Geometry check sheet. Reference: drawing and pictorial views, mm from the part's lowest x, y, z. A direction names the side the tool comes from. Coordinates: 2 decimals unless noted, no trailing zeros. Loops run counter-clockwise (first coordinate to the right, second up) from the corner with the lowest first, then second, coordinate; pieces in that order, holes last.
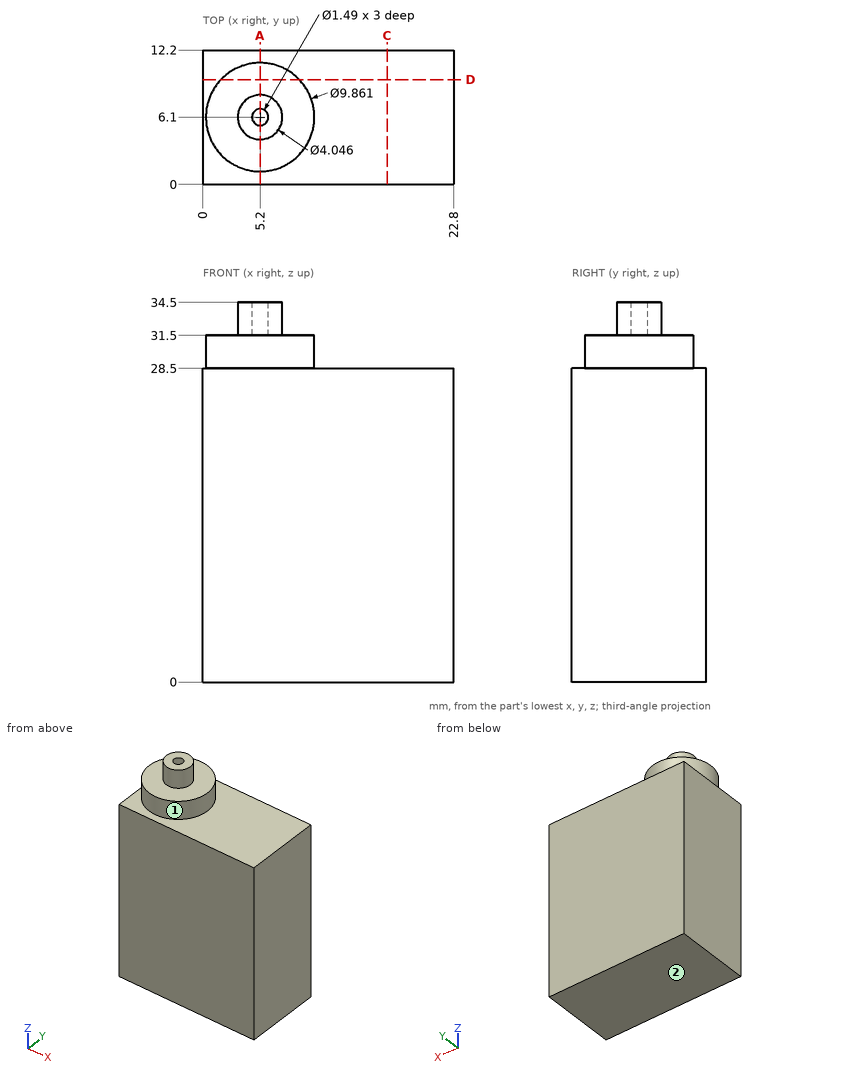
1) Access from +Z, -Z, +X, -X, +Y, -Y to the whole of each face (thin tool, end or side, straight path). Record for the marked faces 1 and 2.
Data:
face 1: +Z
face 2: -Z, +X, -X, +Y, -Y
2) Section check C-C on x = 16.75. Record the cut outline in (y, z).
Data:
outline: (0, 0) - (12.2, 0) - (12.2, 28.5) - (0, 28.5) - close
3) Section check A-A on x = 5.2. Record the cut outline in (y, z) (1 decimal), and give its area (3 significant figures).
Data:
outline: (0, 0) - (12.2, 0) - (12.2, 28.5) - (11, 28.5) - (11, 31.5) - (8.1, 31.5) - (8.1, 34.5) - (6.8, 34.5) - (6.8, 31.5) - (5.4, 31.5) - (5.4, 34.5) - (4.1, 34.5) - (4.1, 31.5) - (1.2, 31.5) - (1.2, 28.5) - (0, 28.5) - close
area: 385 mm2
4) Depth check by flat-ended pin: pin 1 (1.5 mm diameter, centred on x = 18, y = 6, fed in from +Z). Enter the tip coordinate at first touch or a pass-through.
Data:
pin 1: stops at z = 28.5
5) Material ranges on probe 1 along Z at (x, y) = (17.5, 11.25); probe 2 along Z at (x, y) = (2, 9.5); probe 3 along X at (y, z) = (7.5, 29.5), recorded low to high.
Data:
probe 1: z = 0 to 28.5
probe 2: z = 0 to 31.5
probe 3: x = 0.47 to 9.93
6) Section check D-D on y = 9.5. Record the cut outline in (x, z), and give its area (3 significant figures).
Data:
outline: (0, 0) - (22.8, 0) - (22.8, 28.5) - (8.77, 28.5) - (8.77, 31.5) - (1.63, 31.5) - (1.63, 28.5) - (0, 28.5) - close
area: 671 mm2
